Read the model definition and answer for the solid it produces. Units are mm, in the model's axes. Face numbers are marked on the shaded views. A direction names the side the tool comes from. Coordinates: 2 decimals unless noted, no trailing zeros. Write each loop counter-clockwise with the first axis right and the second up, starting at its lowest first coordinate (ties: lowest second). Pieces come first, ordered by that corner, then holes. Notation, with made-up numbers: (40.25, 78.5) -> (85.25, 78.5) arc R15 ccw to (85.25, 83.5) -> close; hole circle Ø6 at (53.25, 14.25). An arc over 180 degrees is marked (long way). Answer as a JSON object with one key per item and string values. Group by question number.
(1) Which of the six approach directions +Z, -Z, +X, -X, +Y, -Y give full straight-line access (tool end or side, diameter ignored) to the marked faces 4, 5, 6 and 7?
(2) Find section C-C (y = 0). Give the vertices of the cut face in (x, z), then the cut area to 3 significant figures.
(3) Straight lines are drawn through the part: L1, parallel to Y at x = 0, z = -44; L2, parallel to Z at x = 18.5, y = 0; L3, parallel to Y at x = 29.5, z = -36. For each, find the intervals that lie inside material, in ascending order.
(4) Find section B-B (x = 6). Give the vertices of the cut face in (y, z).
(5) Flat-ended cylindrical pins translate along their axes: P1, Ø4, axis at x = 13.5, z = -67.5, coming from the +Y side; P2, Ø12, axis at y = 0, z = -30, coming from the +X side; P3, Ø9, axis at x = -12, z = -4.5, coming from the -Y side. Find the tip coordinate at first contact, or state that the pin passes through.
(6) Find section A-A (z = -67). Give the vertices of the cut face in (x, y).
(7) For a pull along Z with two mould halves and no side action, classify the marked faces 1, 2 and 3 as +Z half, -Z half, draft (parallel to the pull), parting line (faces both ways), or undercut.
(8) Find section D-D (y = 12). Give the vertices of the cut face in (x, z), then the cut area to 3 significant figures.
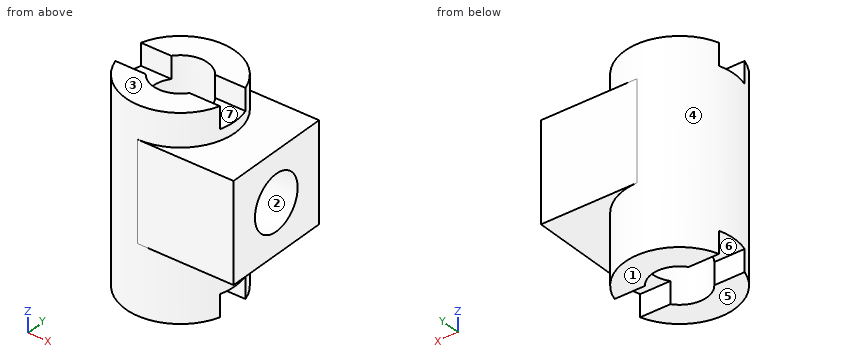
Autodesk Inventor part; units mm, degrees
ref_plane "Płaszczyzna konstrukcyjna1" through (35, -6, 0) normal (1, 0, 0) x (0, 0, -1)
ref_plane "Płaszczyzna konstrukcyjna2" through (35, -6, 0) normal (1, 0, 0) x (0, 0, -1)
ref_plane "YZ Plane" through (0, 0, 0) normal (1, 0, 0) x (0, 1, 0)
sketch "Szkic1" plane through (0, 0, 0) normal (0, 0, 1) x (1, 0, 0)
  circle A0 centre (0, 0) radius 20
  circle A1 centre (0, 0) radius 10
  dimension "d0" = 40
  dimension "d1" = 20
extrude "Wyciągnięcie proste1" add sketch "Szkic1" against normal blind 73
sketch "Szkic2" plane through (0, 0, 0) normal (0, 0, 1) x (1, 0, 0)
  line L0 (0, 0) -> (0, 6)
  line L1 (0, 6) -> (24.4781, 6)
  line L2 (24.4781, 6) -> (24.4781, -6)
  line L3 (24.4781, -6) -> (-24.6977, -6)
  line L4 (-24.6977, -6) -> (-24.6977, 6)
  line L5 (-24.6977, 6) -> (0, 6)
  dimension "d4" = 6
  dimension "d5" = 12
extrude "Wyciągnięcie proste2" cut sketch "Szkic2" against normal blind 8
sketch "Szkic3" plane through (0, 0, -73) normal (0, 0, -1) x (-1, 0, 0)
  line L0 (0, 0) -> (23.7964, 0)
  line L1 (0, 0) -> (26.8721, 0)
  line L2 (26.8721, 0) -> (26.8721, 6)
  line L3 (26.8721, 6) -> (-29.6241, 6)
  line L4 (-29.6241, 6) -> (-29.6241, -6)
  line L5 (-29.6241, -6) -> (26.8721, -6)
  line L6 (26.8721, -6) -> (26.8721, 0)
  dimension "d8" = 6
  dimension "d9" = 12
extrude "Wyciągnięcie proste3" cut sketch "Szkic3" against normal blind 8
ref_plane "Płaszczyzna konstrukcyjna1" through (35, -6, 0) normal (1, 0, 0) x (0, 0, -1)
sketch "Szkic5" plane through (35, -6, 0) normal (1, 0, 0) x (0, 0, -1)
  point P0 (0, 6)
ref_plane "Płaszczyzna konstrukcyjna2" through (35, -6, 0) normal (1, 0, 0) x (0, 0, -1)
sketch "Szkic6" plane through (35, -6, 0) normal (1, 0, 0) x (0, 0, -1)
  line L0 (12, 0) -> (12, 2)
  line L1 (12, 2) -> (12, 26)
  line L2 (0, 26) -> (73, 26)
  line L3 (12, 26) -> (48, 26)
  line L4 (48, 26) -> (48, -14)
  line L5 (0, -14) -> (73, -14)
  line L6 (12, -14) -> (12, 2)
  line L7 (12, 0) -> (0, 0)
  point P0 (0, 6)
  dimension "d16" = 36
extrude "Wyciągnięcie proste5" add sketch "Szkic6" against normal blind 35
sketch "Szkic7" plane through (0, 0, -12) normal (0, 0, 1) x (1, 0, 0)
  circle A0 centre (0, 0) radius 10
  dimension "d19" = 20
extrude "Wyciągnięcie proste6" cut sketch "Szkic7" against normal blind 65
sketch "Szkic8" plane through (35, -6, 0) normal (1, 0, 0) x (0, 0, -1)
  line L0 (12, 26) -> (12, -14)
  circle A0 centre (30, 6) radius 10
  point P0 (0, 6)
  dimension "d24" = 20
extrude "Wyciągnięcie proste7" cut sketch "Szkic8" against normal blind 35
Results below:
{
 "1": {"face 4": "none", "face 5": "-Z, +X, -X, +Y, -Y", "face 6": "-Z, +X, -X", "face 7": "+Z, +X, -X"},
 "2": {"outline": "(-20, -65) -> (-10, -65) -> (-10, -8) -> (-20, -8) -> close; (10, -65) -> (20, -65) -> (20, -48) -> (35, -48) -> (35, -40) -> (10, -40) -> close; (10, -20) -> (35, -20) -> (35, -12) -> (20, -12) -> (20, -8) -> (10, -8) -> close", "area": "1,180 mm2"},
 "3": {"L1": "y = -20 to -10, 10 to 20", "L2": "z = -65 to -40, -20 to -8", "L3": "y = -20 to -8, 8 to 20"},
 "4": {"outline": "(-20, -48) -> (-19.08, -48) -> (-19.08, -73) -> (-8, -73) -> (-8, -36) arc R10 cw to (-8, -24) -> (-8, 0) -> (-19.08, 0) -> (-19.08, -12) -> (-20, -12) -> close; (8, -73) -> (19.08, -73) -> (19.08, -48) -> (20, -48) -> (20, -12) -> (19.08, -12) -> (19.08, 0) -> (8, 0) -> (8, -24) arc R10 cw to (8, -36) -> close"},
 "5": {"P1": "stops at y = 16.36", "P2": "stops at x = -8", "P3": "stops at y = -18.54"},
 "6": {"outline": "(-19.08, -6) arc R20 ccw to (19.08, -6) -> (8, -6) arc R10 cw to (-8, -6) -> close; (-19.08, 6) -> (-8, 6) arc R10 cw to (8, 6) -> (19.08, 6) arc R20 ccw to start"},
 "7": {"face 1": "-Z half", "face 2": "undercut", "face 3": "+Z half"},
 "8": {"outline": "(-16, -73) -> (16, -73) -> (16, -48) -> (35, -48) -> (35, -12) -> (16, -12) -> (16, 0) -> (-16, 0) -> close", "area": "3,020 mm2"}
}
